Here's how the part is built. I have some questions about the finished solid (model axes, mm). Coordinates: 2 decimals unless noted, no trailing zeros. Loops run counter-clockwise (first coordinate to the right, second up) from the corner with the lowest first, then second, coordinate; pieces in that order, holes last. Notation, with made-up numbers: M -25.75,-24.75 L 19.25,-24.75 A28 cw 19.25,-2.75 Z; hole C 28,87 d10. An arc over 180 degrees is marked long. Use CSV: the item, a comma, the result in double quotes. Start each with the question number.
Q1. If we section it at B-B (z = 1): State how many separate pieces and enclosed holes the cut face has, and give its area (3 significant figures).
Q2. Please list where these lines run through material, in increasing order: probe 1 along X at (y, z) = (7.5, 3.1); probe 2 along Y at (x, z) = (-26, 2.1); probe 3 along X at (y, z) = (9.75, 2.05). Write a range as [from, to].
Q3. If we section it at C-C (x = -4.5): Please give me the cut outline in (y, z), and give its area (3 significant figures).
Q4. For pin 1 Ø1.5 at (y, z) = (7.5, 2) entering from -X; pin 2 Ø3 at (y, z) = (8.5, 1) entering from -X; pin 3 Ø1.2 at (y, z) = (7, 3.5) entering from +X, each with a flat end and sliding along its axis, tell me the tip position at first contact or that it passes through.
Q5. If we section it at A-A (y = 6.5): Please give me the cut outline in (x, z), and give its area (3 significant figures).
from build123d import *

# Parameters (mm, degrees)
F1_DEPTH = 5
F2_R     = 2
F3_R     = 1


with BuildPart() as f1:
    # F0 (on Top) → F1 (new body)
    with BuildSketch(Plane.XY):
        Polygon((0, 3), (0, 0), (62, 0), (62, 3), (55, 3), (55, 7), (51, 7), (51, 3), (2, 3), (2, 7), (0, 7), align=None)
    extrude(amount=F1_DEPTH)

    # F2
    f2_edges = [f1.edges().sort_by_distance(p)[0] for p in [
        (55, 3, 2.5),
    ]]
    fillet(f2_edges, radius=F2_R)

    # F3
    f3_edges = [f1.edges().sort_by_distance(p)[0] for p in [
        (51, 3, 2.5),
        (2, 3, 2.5),
    ]]
    fillet(f3_edges, radius=F3_R)

    # F4: F1 across face


with BuildPart() as f1_1:
    add(f1.part)
    add(f1.part.mirror(Plane(origin=(0, 3.5, 2.5), x_dir=(0, -1, 0), z_dir=(-1, 0, 0))))

    # F5: F1 across face


with BuildPart() as f1_2:
    add(f1_1.part)
    add(f1_1.part.mirror(Plane(origin=(0, 7, 2.5), x_dir=(-1, 0, 0), z_dir=(0, 1, 0))))


solid = f1_2.part
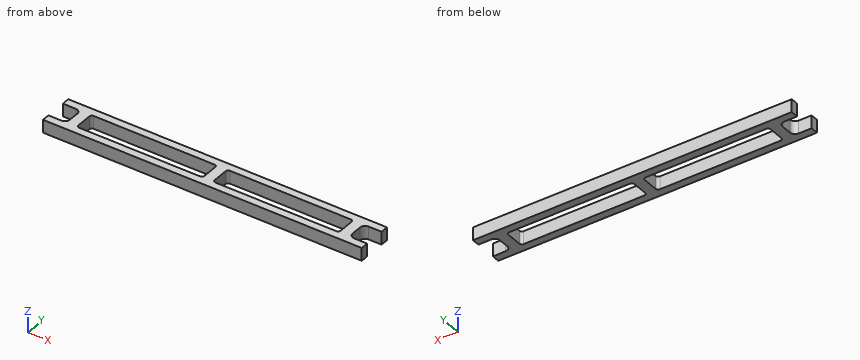
Results below:
1,separate pieces,"1"
1,enclosed holes,"2"
1,area,"845 mm^2"
2,probe 1,"[-55, -51], [-2, 2], [51, 55]"
2,probe 2,"[0, 3], [11, 14]"
2,probe 3,"[-55.15, -51], [-2, 2], [51, 55.15]"
3,outline,"M 0,0 L 3,0 L 3,5 L 0,5 Z; M 11,0 L 14,0 L 14,5 L 11,5 Z"
3,area,"30.0 mm^2"
4,pin 1,"x = -55"
4,pin 2,"x = -55.27"
4,pin 3,"x = 55"
5,outline,"M -55,0 L -51,0 L -51,5 L -55,5 Z; M -2,0 L 2,0 L 2,5 L -2,5 Z; M 51,0 L 55,0 L 55,5 L 51,5 Z"
5,area,"60.0 mm^2"
